Design review of the part built by this model. Coordinates are the model's own, in mm. Face numbers are marked on the shaded views. Coordinates: 2 decimals unless noted, no trailing zeros. Write each loop counter-clockwise with the first axis right and the second up, starting at its lowest first coordinate (ties: lowest second). Pieces come first, ordered by that corner, then holes. Notation, with made-up numbers: (-28, 3) -> (20, 3) arc R19 cw to (20, 40) -> close; hole circle Ø6 at (-34, 87). An arc over 180 degrees is marked (long way). Answer in a Markdown table with one row per item. Add a question column.
Item 1: To check wall thickness, follow line 1 (Y direction, x = 4, z = 0); line 2 (Y direction, x = 5, z = 18); line 3 (Z direction, x = 1.75, y = -33.5). State the ranges of each line that lie inside material, in increasing order.
Item 2: Take a section at B-B, the plane y = 0. Write out the cut boundary in (x, z).
Item 3: Take a section at D-D, the plane z = 37. Write out the cut boundary in (x, y).
Item 4: Clearance check with flat-ended pins moving along their axes: P1, Ø4, axis at x = 4.5, z = -22.5, coming from the +Y side; P2, Ø3, axis at x = 2.5, y = -13, coming from the -Z side; P3, Ø4, axis at x = 4.5, z = 17, coming from the +Y side. State where each tip first meets the part, or that it passes through.
Item 5: Draft analysis for pull direction Y (two halves, no side actions). For the marked faces 1, 2 and 3, state which applies: released by +Y, released by -Y, zero draft, split by the parting line, or undercut.
Item 6: Take a section at A-A, the plane z = 0. Write out the cut boundary in (x, y), and give its area (3 significant figures).
Item 7: Take a section at C-C, the plane y = -25. Write out the cut boundary in (x, z).
from build123d import *

# Parameters (mm, degrees)
SKETCH1_R           = 4
SKETCH1_R_2         = 17.5
BOSS_EXTRUDE1_DEPTH = 8
CUT_EXTRUDE1_REACH  = 95
SKETCH2_W           = 20
SKETCH2_H           = 8
SKETCH2_W_2         = 8
SKETCH2_H_2         = 10
SKETCH2_W_3         = 7
SKETCH2_H_3         = 4


with BuildPart() as part:
    # Sketch1 → Boss-Extrude1 (new body)
    with BuildSketch(Plane(origin=(0, 0, 0), x_dir=(0, 0, -1), z_dir=(1, 0, 0))):
        with BuildLine():
            Line((-12.5, -62.767427859), (-12.5, -67))
            Line((-12.5, -67), (12.5, -67))
            Line((12.5, -67), (12.5, -62.767427859))
            ThreePointArc((12.5, -62.767427859), (0, 64), (-12.5, -62.767427859))
        make_face()
        with Locations((0, 50)):
            Circle(SKETCH1_R, mode=Mode.SUBTRACT)
        with Locations((43.301270189, -25)):
            Circle(SKETCH1_R, mode=Mode.SUBTRACT)
        with Locations((-43.301270189, -25)):
            Circle(SKETCH1_R, mode=Mode.SUBTRACT)
        with Locations((-26.1, 0)):
            Circle(SKETCH1_R_2, mode=Mode.SUBTRACT)
        with Locations(Location((26.1, 0, 0), (0, 0, 180))):
            Circle(SKETCH1_R_2, mode=Mode.SUBTRACT)
    extrude(amount=BOSS_EXTRUDE1_DEPTH)

    # Sketch2 → Cut-Extrude1 (cut, up to next)
    with BuildSketch(Plane.ZY, mode=Mode.PRIVATE) as cut_extrude1_sk1:
        with Locations((20, -31.5)):
            Rectangle(SKETCH2_W, SKETCH2_H)
    cut_extrude1_tool1 = extrude(cut_extrude1_sk1.sketch, amount=-CUT_EXTRUDE1_REACH, mode=Mode.PRIVATE) & part.part
    # Sketch2 → Cut-Extrude1 (cut, up to next)
    with BuildSketch(Plane.ZY, mode=Mode.PRIVATE) as cut_extrude1_sk2:
        with Locations((-20, -31.5)):
            Rectangle(SKETCH2_W, SKETCH2_H)
    cut_extrude1_tool2 = extrude(cut_extrude1_sk2.sketch, amount=-CUT_EXTRUDE1_REACH, mode=Mode.PRIVATE) & part.part
    # Sketch2 → Cut-Extrude1 (cut, up to next)
    with BuildSketch(Plane.ZY, mode=Mode.PRIVATE) as cut_extrude1_sk3:
        with Locations((20, 31.5)):
            Rectangle(SKETCH2_W, SKETCH2_H)
    cut_extrude1_tool3 = extrude(cut_extrude1_sk3.sketch, amount=-CUT_EXTRUDE1_REACH, mode=Mode.PRIVATE) & part.part
    # Sketch2 → Cut-Extrude1 (cut, up to next)
    with BuildSketch(Plane.ZY, mode=Mode.PRIVATE) as cut_extrude1_sk4:
        with Locations((-20, 31.5)):
            Rectangle(SKETCH2_W, SKETCH2_H)
    cut_extrude1_tool4 = extrude(cut_extrude1_sk4.sketch, amount=-CUT_EXTRUDE1_REACH, mode=Mode.PRIVATE) & part.part
    # Sketch2 → Cut-Extrude1 (cut, up to next)
    with BuildSketch(Plane.ZY, mode=Mode.PRIVATE) as cut_extrude1_sk5:
        with Locations((0, 22.5)):
            Rectangle(SKETCH2_W_2, SKETCH2_H_2)
    cut_extrude1_tool5 = extrude(cut_extrude1_sk5.sketch, amount=-CUT_EXTRUDE1_REACH, mode=Mode.PRIVATE) & part.part
    # Sketch2 → Cut-Extrude1 (cut, up to next)
    with BuildSketch(Plane.ZY, mode=Mode.PRIVATE) as cut_extrude1_sk6:
        with Locations((0, -22.5)):
            Rectangle(SKETCH2_W_2, SKETCH2_H_2)
    cut_extrude1_tool6 = extrude(cut_extrude1_sk6.sketch, amount=-CUT_EXTRUDE1_REACH, mode=Mode.PRIVATE) & part.part
    # Sketch2 → Cut-Extrude1 (cut, up to next)
    with BuildSketch(Plane.ZY, mode=Mode.PRIVATE) as cut_extrude1_sk7:
        with Locations((9, -65)):
            Rectangle(SKETCH2_W_3, SKETCH2_H_3)
    cut_extrude1_tool7 = extrude(cut_extrude1_sk7.sketch, amount=-CUT_EXTRUDE1_REACH, mode=Mode.PRIVATE) & part.part
    # Sketch2 → Cut-Extrude1 (cut, up to next)
    with BuildSketch(Plane.ZY, mode=Mode.PRIVATE) as cut_extrude1_sk8:
        with Locations((-9, -65)):
            Rectangle(SKETCH2_W_3, SKETCH2_H_3)
    cut_extrude1_tool8 = extrude(cut_extrude1_sk8.sketch, amount=-CUT_EXTRUDE1_REACH, mode=Mode.PRIVATE) & part.part
    add(cut_extrude1_tool1.solids().sort_by_distance((0, -31.5, 20))[0], mode=Mode.SUBTRACT)
    add(cut_extrude1_tool2.solids().sort_by_distance((0, -31.5, -20))[0], mode=Mode.SUBTRACT)
    add(cut_extrude1_tool3.solids().sort_by_distance((0, 31.5, 20))[0], mode=Mode.SUBTRACT)
    add(cut_extrude1_tool4.solids().sort_by_distance((0, 31.5, -20))[0], mode=Mode.SUBTRACT)
    add(cut_extrude1_tool5.solids().sort_by_distance((0, 22.5, 0))[0], mode=Mode.SUBTRACT)
    add(cut_extrude1_tool6.solids().sort_by_distance((0, -22.5, 0))[0], mode=Mode.SUBTRACT)
    add(cut_extrude1_tool7.solids().sort_by_distance((0, -65, 9))[0], mode=Mode.SUBTRACT)
    add(cut_extrude1_tool8.solids().sort_by_distance((0, -65, -9))[0], mode=Mode.SUBTRACT)


solid = part.part
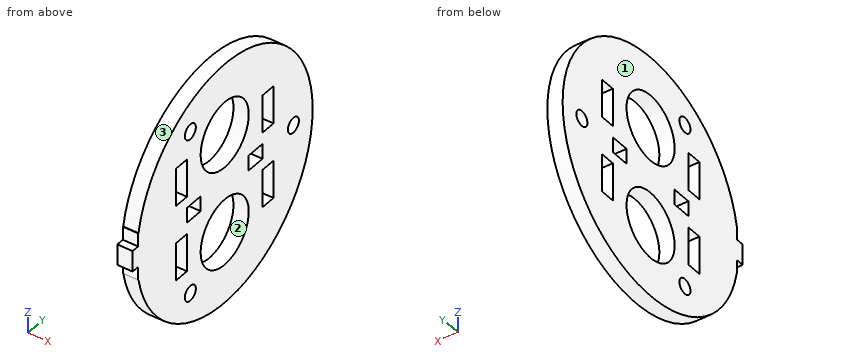
Answers:
| question | item | result |
|---|---|---|
| 1 | line 1 | y = -67 to -27.5, -17.5 to 17.5, 27.5 to 46, 54 to 64 |
| 1 | line 2 | y = -61.42 to -35.5, -27.5 to -15.51, 15.51 to 27.5, 35.5 to 61.42 |
| 1 | line 3 | z = -54.53 to -30, -10 to 10, 30 to 54.53 |
| 2 | outline | (0, -64) -> (8, -64) -> (8, -43.6) -> (0, -43.6) -> close; (0, -8.6) -> (8, -8.6) -> (8, 8.6) -> (0, 8.6) -> close; (0, 43.6) -> (8, 43.6) -> (8, 64) -> (0, 64) -> close |
| 3 | outline | (0, -52.22) -> (8, -52.22) -> (8, -13.69) -> (0, -13.69) -> close; (0, 13.69) -> (8, 13.69) -> (8, 52.22) -> (0, 52.22) -> close |
| 4 | P1 | stops at y = 60.63 |
| 4 | P2 | stops at z = -62.96 |
| 4 | P3 | stops at y = 62.22 |
| 5 | face 1 | zero draft |
| 5 | face 2 | undercut |
| 5 | face 3 | split by the parting line |
| 6 | outline | (0, -67) -> (8, -67) -> (8, -27.5) -> (0, -27.5) -> close; (0, -17.5) -> (8, -17.5) -> (8, 17.5) -> (0, 17.5) -> close; (0, 27.5) -> (8, 27.5) -> (8, 46) -> (0, 46) -> close; (0, 54) -> (8, 54) -> (8, 64) -> (0, 64) -> close |
| 6 | area | 824 mm^2 |
| 7 | outline | (0, -58.92) -> (8, -58.92) -> (8, -47.3) -> (0, -47.3) -> close; (0, -39.3) -> (8, -39.3) -> (8, -4) -> (0, -4) -> close; (0, 4) -> (8, 4) -> (8, 39.3) -> (0, 39.3) -> close; (0, 47.3) -> (8, 47.3) -> (8, 58.92) -> (0, 58.92) -> close |
